Part print with two shaded views. Sizes in mm from the minimum x, y, z corner. A direction names the side the tool comes from. Round coordinates to 2 decimals unless told otherwise and drop trailing zeros. Loops run counter-clockwise (first coordinate to the right, second up) from the corner with the lowest first, then second, coordinate; pieces in that order, holes last. Notation, with made-up numbers: M 46,17 L 97,17 A27 cw 97,40 Z; hole C 0,77 d5. An arc over 180 degrees is marked long. Answer as CSV lines item,"result". Start each with the question number.
Item 1: Which spindle directions (+Z, -Z, +X, -X, +Y, -Y) get a long thin tool onto all of the face, cutting with end or side? Do the marked faces 5 and 6. Say none if no direction does.
Item 2: Mould opens along Z. For the marked faces 1, 2, 3 and 4 say: pulls with the +Z half, pulls with the -Z half, needs draft (parallel to the pull), parting line crosses it, or undercut.
Item 3: Drop a flat-ended pin along its axis: pin 1 Ø1 at (x, y) = (8.5, 10.5) entering from -Z. Give the stop position or say it passes through.
Item 4: Band-saw the part on B-B (z = 3). Give the cut face in (x, y), and give its area (3 significant figures).
Item 5: Band-saw the part on D-D (z = 7). Give the cut face in (x, y), and give its area (3 significant figures).
Item 6: Band-saw the part on C-C (y = 11.5). Give the cut face in (x, z).
Item 7: Band-saw the part on A-A (x = 18). Give the cut face in (y, z), and give its area (3 significant figures).
Item 8: Wall check: line 1 (Y direction, x = 17.5, z = 3.5); line 2 (Z direction, x = 3.5, y = 10.75); line 3 (X direction, y = 8.5, z = 3.5). Give the ranges that are in metal, low to high.
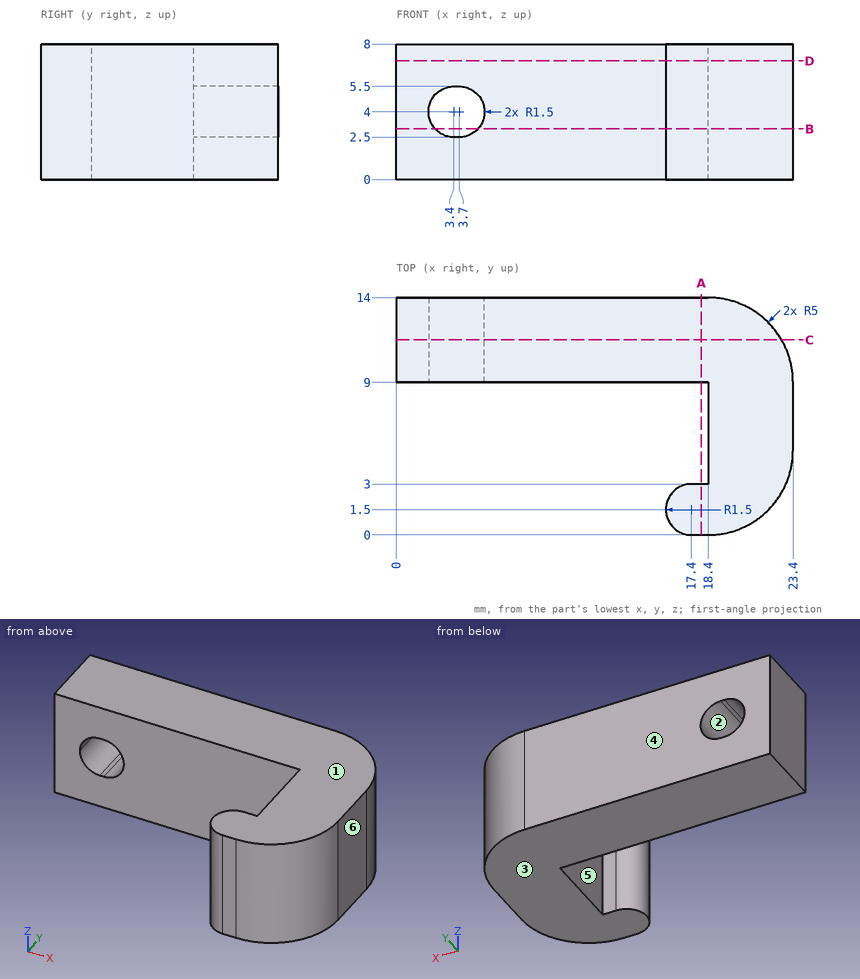
Answer block:
1,face 5,"+Z, -Z, -X"
1,face 6,"+Z, -Z, +X, +Y, -Y"
2,face 1,"pulls with the +Z half"
2,face 2,"undercut"
2,face 3,"pulls with the -Z half"
2,face 4,"needs draft"
3,pin 1,"stops at z = 0"
4,outline,"M 0,9 L 2.28,9 L 2.28,14 L 0,14 Z; M 4.82,9 L 18.4,9 L 18.4,3 L 17.4,3 A1.5 ccw 17.4,0 L 18.4,0 A5 ccw 23.4,5 L 23.4,9 A5 ccw 18.4,14 L 4.82,14 Z"
4,area,"145 mm^2"
5,outline,"M 0,9 L 18.4,9 L 18.4,3 L 17.4,3 A1.5 ccw 17.4,0 L 18.4,0 A5 ccw 23.4,5 L 23.4,9 A5 ccw 18.4,14 L 0,14 Z"
5,area,"158 mm^2"
6,outline,"M 0,0 L 22.73,0 L 22.73,8 L 0,8 Z; hole M 3.4,2.5 L 3.7,2.5 A1.5 ccw 3.7,5.5 L 3.4,5.5 A1.5 ccw Z"
7,outline,"M 0,0 L 3,0 L 3,8 L 0,8 Z; M 9,0 L 14,0 L 14,8 L 9,8 Z"
7,area,"64.0 mm^2"
8,line 1,"y = 0 to 3, 9 to 14"
8,line 2,"z = 0 to 2.5, 5.5 to 8"
8,line 3,"x = 18.4 to 23.4"
